Geometry: final body of the model. Coordinates: model frame, mm. Face numbers are marked on the shaded views. A direction names the side the tool comes from. Coordinates: 2 decimals unless noted, no trailing zeros. Write each loop counter-clockwise with the first axis right and the second up, starting at its lowest first coordinate (ties: lowest second). Pieces come first, ordered by that corner, then holes. Notation, with made-up numbers: (25.5, 64.25) -> (82.5, 64.25) arc R24 ccw to (82.5, 99.25) -> close; hole circle Ø4 at (-33.5, 51.5). An arc over 180 degrees is marked (long way). One line per item, written item: value.
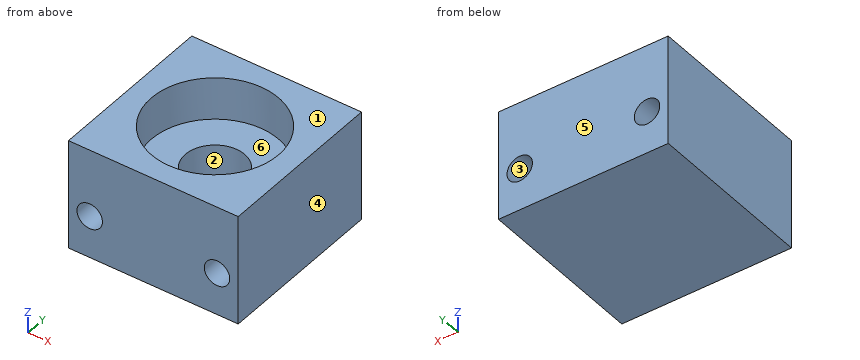
```python
from build123d import *

# Parameters (mm, degrees)
ESQUISSE1_W             = 20
ESQUISSE1_H             = 20
BOSS_EXTRU_1_DEPTH      = 13
ESQUISSE2_R             = 7.5
ENL_V_MAT_EXTRU_1_DEPTH = 5
ESQUISSE3_R             = 3.5
ENL_V_MAT_EXTRU_2_DEPTH = 5
ESQUISSE4_R             = 1.5
ENL_V_MAT_EXTRU_3_DEPTH = 21


with BuildPart() as part:
    # Esquisse1 → Boss.-Extru.1 (new body)
    with BuildSketch(Plane.XY):
        with Locations((10, 10)):
            Rectangle(ESQUISSE1_W, ESQUISSE1_H)
    extrude(amount=BOSS_EXTRU_1_DEPTH)

    # Esquisse2 → Enlèv. mat.-Extru.1 (cut)
    with BuildSketch(Plane.XY.offset(13)):
        with Locations((10, 10)):
            Circle(ESQUISSE2_R)
    extrude(amount=-ENL_V_MAT_EXTRU_1_DEPTH, mode=Mode.SUBTRACT)

    # Esquisse3 → Enlèv. mat.-Extru.2 (cut)
    with BuildSketch(Plane.XY.offset(8)):
        with Locations((10, 10)):
            Circle(ESQUISSE3_R)
    extrude(amount=-ENL_V_MAT_EXTRU_2_DEPTH, mode=Mode.SUBTRACT)

    # Esquisse4 → Enlèv. mat.-Extru.3 (cut, through all)
    with BuildSketch(Plane(origin=(0, 20, 0), x_dir=(1, 0, 0), z_dir=(0, 1, 0))):
        with Locations((17.5, -5)):
            Circle(ESQUISSE4_R)
        with Locations((2.5, -5)):
            Circle(ESQUISSE4_R)
    extrude(amount=-ENL_V_MAT_EXTRU_3_DEPTH, mode=Mode.SUBTRACT)


solid = part.part
```
(1) Reachability of the marked faces 1 and 2 from +Z, -Z, +X, -X, +Y, -Y: full face, straight path, thin tool, end or side. Return the list, or none.
Responses:
face 1: +Z, +X, -X, +Y, -Y
face 2: +Z
(2) Section D-D (x = 10). Return the cut outline in (y, z).
Responses:
outline: (0, 0) -> (20, 0) -> (20, 13) -> (17.5, 13) -> (17.5, 8) -> (13.5, 8) -> (13.5, 3) -> (6.5, 3) -> (6.5, 8) -> (2.5, 8) -> (2.5, 13) -> (0, 13) -> close
(3) Section C-C (x = 2.75). Return the cut outline in (y, z).
Responses:
outline: (0, 0) -> (20, 0) -> (20, 3.52) -> (0, 3.52) -> close; (0, 6.48) -> (20, 6.48) -> (20, 13) -> (11.92, 13) -> (11.92, 8) -> (8.08, 8) -> (8.08, 13) -> (0, 13) -> close
(4) Section A-A (y = 10). Return the cut outline in (x, z), then the cut area to 3 significant figures.
Responses:
outline: (0, 0) -> (20, 0) -> (20, 13) -> (17.5, 13) -> (17.5, 8) -> (13.5, 8) -> (13.5, 3) -> (6.5, 3) -> (6.5, 8) -> (2.5, 8) -> (2.5, 13) -> (0, 13) -> close; hole circle Ø3 at (2.5, 5); hole circle Ø3 at (17.5, 5)
area: 136 mm2
(5) Line query: line 1 (X direction, y = 4.25, z = 5); line 2 (Z direction, x = 2.5, y = 9); line 3 (X direction, y = 4.25, z = 12.5). Output: solid intervals per line, ascending. Write a range as [from, to].
Responses:
line 1: x = [0, 1], [4, 16], [19, 20]
line 2: z = [0, 3.5], [6.5, 13]
line 3: x = [0, 5.18], [14.82, 20]
(6) Section B-B (z = 4.5). Return the cut outline in (x, y), then the cut area to 3 significant figures.
Responses:
outline: (0, 0) -> (1.09, 0) -> (1.09, 20) -> (0, 20) -> close; (3.91, 0) -> (16.09, 0) -> (16.09, 20) -> (3.91, 20) -> close; (18.91, 0) -> (20, 0) -> (20, 20) -> (18.91, 20) -> close; hole circle Ø7 at (10, 10)
area: 248 mm2
(7) First-contact query: pin 1 (9 mm diameter, centred on x = 10, y = 10, fed in from -Z); pin 2 (4.5 mm diameter, centred on x = 7.5, y = 9, fed in from +Z). Flat tips, straight axial feed; report the tip coordinate or a pass-through.
Responses:
pin 1: stops at z = 0
pin 2: stops at z = 8
(8) Pull-direction query (X, two-part tool) for the marked faces 3, 4, 5 and 6; classes: released by +X, released by -X, zero draft, split by the parting line, or undercut.
Responses:
face 3: undercut
face 4: released by +X
face 5: zero draft
face 6: undercut
